```python
from build123d import *

# Parameters (mm, degrees)
BOSS_EXTRUDE2_DEPTH = 6.35
SKETCH2_R           = 3.175
CUT_EXTRUDE1_DEPTH  = 7.35
SKETCH5_R           = 4.6625
BOSS_EXTRUDE3_DEPTH = 12.7
SKETCH6_W           = 177.8
SKETCH6_H           = 6.35
CUT_EXTRUDE2_DEPTH  = 3.175
SKETCH7_R           = 2.286
CUT_EXTRUDE3_DEPTH  = 12.7
SKETCH8_R           = 3.175
CUT_EXTRUDE4_DEPTH  = 20.05


with BuildPart() as part:
    # Sketch1 → Boss-Extrude2 (new body)
    with BuildSketch(Plane(origin=(0, 0, 0), x_dir=(1, 0, 0), z_dir=(0, 1, 0))):
        with BuildLine():
            Line((0, 0), (0, 25.4))
            ThreePointArc((0, 25.4), (3.719743879, 34.380256121), (12.7, 38.1))
            Line((12.7, 38.1), (190.5, 38.1))
            ThreePointArc((190.5, 38.1), (199.480256121, 34.380256121), (203.2, 25.4))
            Line((203.2, 25.4), (203.2, -152.4))
            ThreePointArc((203.2, -152.4), (199.480256121, -161.380256121), (190.5, -165.1))
            Line((190.5, -165.1), (12.7, -165.1))
            ThreePointArc((12.7, -165.1), (3.719743879, -161.380256121), (0, -152.4))
            Line((0, -152.4), (0, -127))
            Line((0, -127), (177.8, -127))
            Line((177.8, -127), (177.8, 0))
            Line((177.8, 0), (0, 0))
        make_face()
    extrude(amount=BOSS_EXTRUDE2_DEPTH)

    # Sketch2 → Cut-Extrude1 (cut, through all)
    with BuildSketch(Plane(origin=(0, 6.35, 0), x_dir=(1, 0, 0), z_dir=(0, 1, 0))):
        with Locations((12.7, 25.4)):
            Circle(SKETCH2_R)
        with Locations((190.5, 25.4)):
            Circle(SKETCH2_R)
        with Locations((190.5, -152.4)):
            Circle(SKETCH2_R)
        with Locations((12.7, -152.4)):
            Circle(SKETCH2_R)
    extrude(amount=-CUT_EXTRUDE1_DEPTH, mode=Mode.SUBTRACT)

    # Sketch5 → Boss-Extrude3 (add)
    with BuildSketch(Plane.XZ):
        with Locations((28.575, 136.525)):
            Circle(SKETCH5_R)
        with Locations((174.625, 136.525)):
            Circle(SKETCH5_R)
        with Locations((174.625, -9.525)):
            Circle(SKETCH5_R)
        with Locations((28.575, -9.525)):
            Circle(SKETCH5_R)
    extrude(amount=BOSS_EXTRUDE3_DEPTH)

    # Sketch6 → Cut-Extrude2 (cut)
    with BuildSketch(Plane(origin=(0, 6.35, 0), x_dir=(1, 0, 0), z_dir=(0, 1, 0))):
        with Locations((88.9, -130.175)):
            Rectangle(SKETCH6_W, SKETCH6_H)
        with Locations((88.9, 3.175)):
            Rectangle(SKETCH6_W, SKETCH6_H)
    extrude(amount=-CUT_EXTRUDE2_DEPTH, mode=Mode.SUBTRACT)

    # Sketch7 → Cut-Extrude3 (cut)
    with BuildSketch(Plane(origin=(0, 6.35, 0), x_dir=(1, 0, 0), z_dir=(0, 1, 0))):
        with Locations((188.214, -101.092)):
            Circle(SKETCH7_R)
        with Locations((188.214, -91.186)):
            Circle(SKETCH7_R)
        with Locations((188.214, -35.814)):
            Circle(SKETCH7_R)
        with Locations((188.214, -25.908)):
            Circle(SKETCH7_R)
    extrude(amount=-CUT_EXTRUDE3_DEPTH, mode=Mode.SUBTRACT)

    # Sketch8 → Cut-Extrude4 (cut, through all)
    with BuildSketch(Plane(origin=(0, 6.35, 0), x_dir=(1, 0, 0), z_dir=(0, 1, 0))):
        with Locations((101.6, 25.527)):
            Circle(SKETCH8_R)
        with Locations((190.627, -63.5)):
            Circle(SKETCH8_R)
        with Locations((101.6, -152.527)):
            Circle(SKETCH8_R)
    extrude(amount=-CUT_EXTRUDE4_DEPTH, mode=Mode.SUBTRACT)


solid = part.part
```
The model under review builds one solid part; all positions refer to its coordinate system, in mm. A direction names the side the tool comes from. Give positions to 0.01 mm unless a question says otherwise; leave off trailing zeros. Write each loop counter-clockwise with the first axis right and the second up, starting at its lowest first coordinate (ties: lowest second). Pieces come first, ordered by that corner, then holes. Notation, with made-up numbers: M 1,35.25 L 26,35.25 A34 cw 26,68.25 Z; hole C 26,-22 d7. An arc over 180 degrees is marked long. Write item = value, one per line. Start each with the question number.
Q1. Mouldability with a two-part tool opening along Z and no side actions: class faces 1 (the face through (199.58, 3.13, 161.28)), 2 (the face through (3.62, 3.13, -34.28)), 3 (the face through (29, -12.7, 137)), 4 (the face through (186.4, 3.2, 27.3)) as released by +Z, released by -Z, zero draft, split by the parting line, or undercut.
Q2. For line 1 (X direction, y = 2.25, z = 152.4) (3 decimals); line 2 (Z direction, x = 101.6, y = 2.25); line 3 (Z direction, x = 175, y = 0.75), list the stretches that pass through material, from the lowest coordinate up.
Q3. Clearance check with flat-ended pins moving along their axes: pin 1 (8.5 mm diameter, centred on x = 190.5, z = -25.4, fed in from -Y); pin 2 (1.9 mm diameter, centred on y = 3, z = 42, fed in from -X); pin 3 (5 mm diameter, centred on x = 63.5, z = 130.5, fed in from +Y) (3 decimals); pin 4 (5 mm diameter, centred on y = 0.5, z = 126.5, fed in from -X). State where each tip first meets the part, or that it passes through.
Q4. We need section A-A (z = 63.5). State the section outline as (x, y) points.
Q5. We need section B-B (x = 101.6). State the section outline as (y, z) points (3 decimals), plus the area to 3 significant figures.
Q6. We need section D-D (y = -5.5). State the section outline as (x, z) points (1 decimal).
Q7. Machinability: for faces 5 (the face through (3.82, 3.13, 161.48)), 6 (the face through (178.932, -6.261, -11.311)), 7 (the face through (88, 3.175, -3)), which of the approach directions +Z, -Z, +X, -X, +Y, -Y give a long, thin tool a straight path to every point of the face, cutting with its end or side? Answer none if there is none.
Q8. We need section C-C (x = 48.5). State the section outline as (y, z) points (3 decimals), plus the area to 3 significant figures.
Result set:
q1.face_1 = released by +Z
q1.face_2 = released by -Z
q1.face_3 = zero draft
q1.face_4 = undercut
q2.line_1 = 0 to 9.525, 15.875 to 98.428, 104.772 to 187.325, 193.675 to 203.2
q2.line_2 = -38.1 to -28.7, -22.35 to 0, 127 to 149.35, 155.7 to 165.1
q2.line_3 = -38.1 to 0, 127 to 165.1
q3.pin_1 = 0
q3.pin_2 = 177.8
q3.pin_3 = 3.175
q3.pin_4 = 0
q4.outline = M 177.8,0 L 187.45,0 L 187.45,6.35 L 177.8,6.35 Z; M 193.8,0 L 203.2,0 L 203.2,6.35 L 193.8,6.35 Z
q5.outline = M 0,-38.1 L 6.35,-38.1 L 6.35,-28.702 L 0,-28.702 Z; M 0,-22.352 L 6.35,-22.352 L 6.35,-6.35 L 3.175,-6.35 L 3.175,0 L 0,0 Z; M 0,127 L 3.175,127 L 3.175,133.35 L 6.35,133.35 L 6.35,149.352 L 0,149.352 Z; M 0,155.702 L 6.35,155.702 L 6.35,165.1 L 0,165.1 Z
q5.area = 363 mm2
q6.outline = C 28.6,-9.5 d9.3; C 28.6,136.5 d9.3; C 174.6,-9.5 d9.3; C 174.6,136.5 d9.3
q7.face_5 = +Z, -X, +Y, -Y
q7.face_6 = -Y
q7.face_7 = -X, +Y
q8.outline = M 0,-38.1 L 6.35,-38.1 L 6.35,-6.35 L 3.175,-6.35 L 3.175,0 L 0,0 Z; M 0,127 L 3.175,127 L 3.175,133.35 L 6.35,133.35 L 6.35,165.1 L 0,165.1 Z
q8.area = 444 mm2
